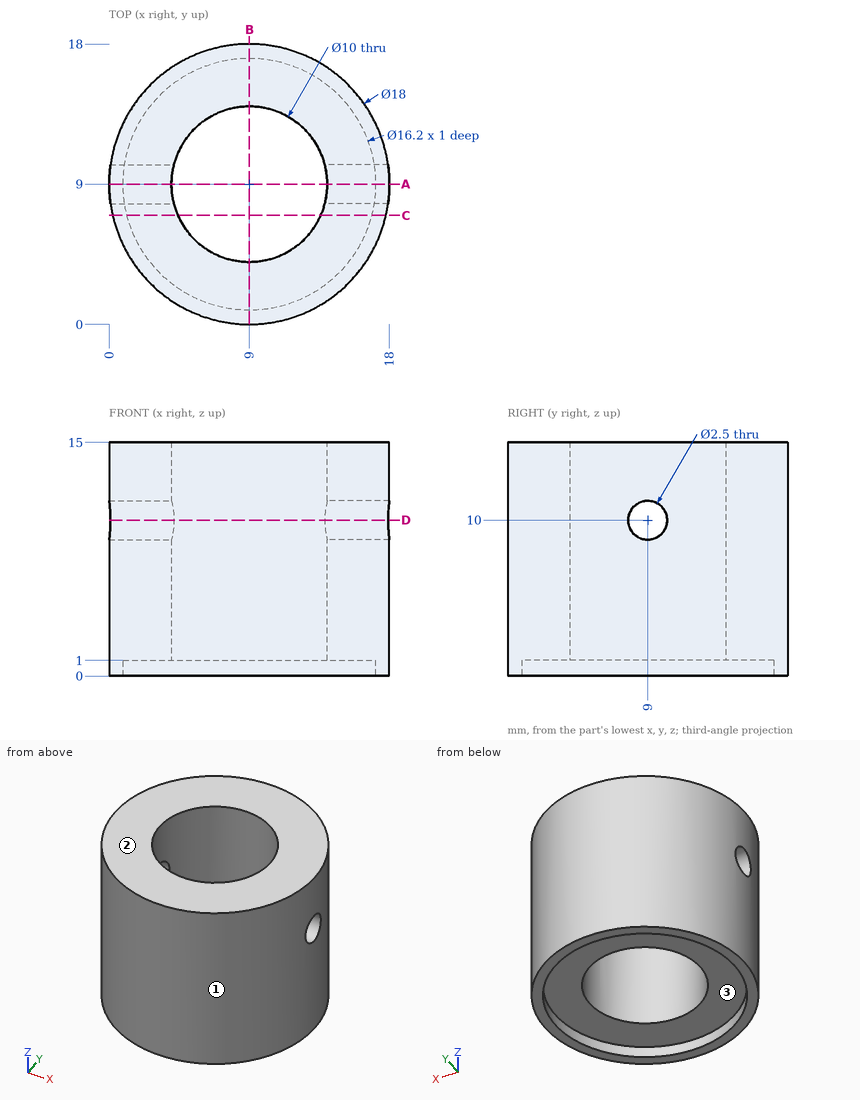
Check sheet for the drawn part. Datum: minimum x, y, z corner. Units: mm. Give positions to 0.01 mm unless a question says otherwise; leave off trailing zeros. Order: outer loops, then holes, each group sorted by start corner. A loop starts at its lowest first (then second) coordinate and runs counter-clockwise, first axis right, second up. Notation, with made-up numbers: (26, 64) - (47, 64) arc R13 ccw to (47, 81) - close; hole circle Ø4 at (19, 75.25). An arc over 180 degrees is marked (long way). Answer in a Markdown table with one row per item. Add a question column.
Q1. Cross-section at D-D, the plane z = 10. Enter the section's corners in (x, y).
Q2. Material ranges on probe 1 along X at (y, z) = (9.25, 7.75); probe 2 along Y at (x, z) = (9, 0.45); probe 3 along Y at (x, z) = (9, 11.75), recorded low to high. Write a range as from..to.
Q3. Cross-section at A-A, the plane y = 9. Enter the section's corners in (x, z).
Q4. Gauge pin test, flat ends, axial feed: pin 1 (2 mm diameter, centred on y = 15.5, z = 6, fed in from -X); pin 2 (6 mm diameter, centred on x = 9, y = 9, fed in from -Z); pin 3 (8 mm diameter, centred on x = 7, y = 8.5, fed in from -Z); pin 4 (1.5 mm diameter, centred on x = 11, z = 2.5, fed in from +Y). Record the tip position at first contact, or that the pin passes through.
Q5. Mould release check, pull along Y, two halves, no side actions. Record for the marked faces 1, 2 and 3: pulls with the +Y half, pulls with the -Y half, needs draft (parallel to the pull), parting line crosses it, or undercut.
Q6. Cross-section at B-B, the plane x = 9. Enter the section's corners in (y, z), then the cut area to 3 significant figures.
Q7. Cross-section at C-C, the plane y = 7. Enter the section's corners in (x, z).
Check values:
| question | item | result |
|---|---|---|
| 1 | outline | (0.09, 7.75) arc R9 ccw to (17.91, 7.75) - (13.84, 7.75) arc R5 cw to (4.16, 7.75) - close; (0.09, 10.25) - (4.16, 10.25) arc R5 cw to (13.84, 10.25) - (17.91, 10.25) arc R9 ccw to start |
| 2 | probe 1 | x = 0..4.01, 13.99..18 |
| 2 | probe 2 | y = 0..0.9, 17.1..18 |
| 2 | probe 3 | y = 0..4, 14..18 |
| 3 | outline | (0, 0) - (0.9, 0) - (0.9, 1) - (4, 1) - (4, 8.75) - (0, 8.75) - close; (0, 11.25) - (4, 11.25) - (4, 15) - (0, 15) - close; (14, 1) - (17.1, 1) - (17.1, 0) - (18, 0) - (18, 8.75) - (14, 8.75) - close; (14, 11.25) - (18, 11.25) - (18, 15) - (14, 15) - close |
| 4 | pin 1 | stops at x = 1.88 |
| 4 | pin 2 | passes through |
| 4 | pin 3 | stops at z = 1 |
| 4 | pin 4 | stops at y = 17.91 |
| 5 | face 1 | parting line crosses it |
| 5 | face 2 | needs draft |
| 5 | face 3 | undercut |
| 6 | outline | (0, 0) - (0.9, 0) - (0.9, 1) - (4, 1) - (4, 15) - (0, 15) - close; (14, 1) - (17.1, 1) - (17.1, 0) - (18, 0) - (18, 15) - (14, 15) - close |
| 6 | area | 114 mm^2 |
| 7 | outline | (0.23, 0) - (1.15, 0) - (1.15, 1) - (4.42, 1) - (4.42, 15) - (0.23, 15) - close; (13.58, 1) - (16.85, 1) - (16.85, 0) - (17.77, 0) - (17.77, 15) - (13.58, 15) - close |
